The listing builds one solid part. Answer for the finished solid, in the listing's coordinates (mm). Face numbers are marked on the shaded views. A direction names the side the tool comes from. Give positions to 0.01 mm unless a question says otherwise; leave off trailing zeros. Write each loop counter-clockwise with the first axis right and the second up, starting at its lowest first coordinate (ties: lowest second). Pieces come first, ordered by that corner, then holes. Notation, with made-up numbers: (2, 62) - (23, 62) arc R23 cw to (23, 98) - close; hole circle Ø8 at (20.5, -23). An arc over 180 degrees is marked (long way). One line per question, with ' | ' between items. Start each with the question number.
1. A cutting plane is placed at D-D (z = 25.5). Determine the outline of the cut face in (x, y), then the cut area to 3 significant figures.
2. A cutting plane is placed at B-B (y = 40.5). Determine the outline of the cut face in (x, z).
3. Find the intervals of material crossed by L1, parallel to Y at x = 84.5, z = 9.5; L2, parallel to Y at x = 20.5, z = 34.5; L3, parallel to X at y = 16, z = 30, in increasing order. Write a range as from..to.
4. For the marked faces 1, 2 and 3, determine the directions among +Z, -Z, +X, -X, +Y, -Y from which every point of the face is accessible in a straight line to the end or side of a thin tool.
5. Given P1, Ø1, axis at x = 29, z = 10.5, coming from the -Y side, flat-ended and moving along its own axis, determine where the tip first touches the part or whether it passes through.
6. A cutting plane is placed at C-C (x = 132). Determine the outline of the cut face in (y, z).
7. The mould has two halves that part along X. Classify the marked faces 4, 5, 6 and 7: +X half, -X half, draft (parallel to the pull), parting line (faces both ways), or undercut.
8. A cutting plane is placed at A-A (x = 60). Determine the outline of the cut face in (y, z).
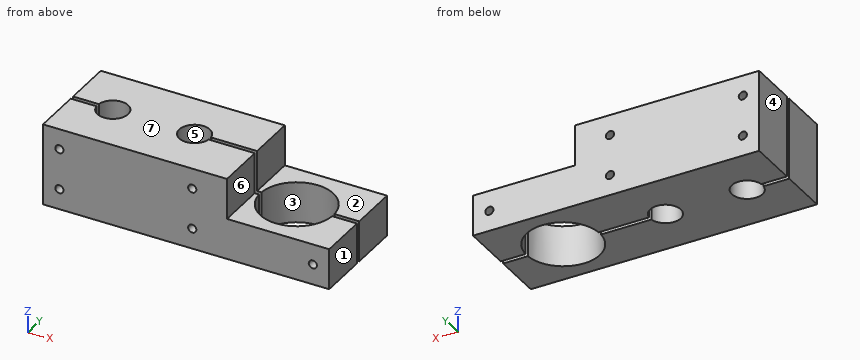
```python
from build123d import *

# Parameters (mm, degrees)
EXTRUDE_1_DEPTH     = 40
SKETCH_8_R          = 2
SKETCH_8_W          = 50
SKETCH_8_H          = 20
CUT_EXTRUDE_1_DEPTH = 50


with BuildPart() as part:
    # Эскиз1 → Бобышка-Вытянуть1 (new body)
    with BuildSketch(Plane.XY):
        with BuildLine():
            Line((67.432912675, 26.000904174), (92.128005404, 26.000904174))
            ThreePointArc((92.128005404, 26.000904174), (110, 42.9), (127.871994596, 26.000904174))
            Line((127.871994596, 26.000904174), (140, 26.000904174))
            Line((140, 26.000904174), (140, 50))
            Line((140, 50), (0, 50))
            Line((0, 50), (0, 26))
            Line((0, 26), (12.566965626, 26))
            ThreePointArc((12.566965626, 26), (27.5, 25), (12.566965626, 24))
            Line((12.566965626, 24), (0, 24))
            Line((0, 24), (0, 0))
            Line((0, 0), (140, 0))
            Line((140, 0), (140, 23.999095826))
            Line((140, 23.999095826), (127.871994596, 23.999095826))
            ThreePointArc((127.871994596, 23.999095826), (110, 7.1), (92.128005404, 23.999095826))
            Line((92.128005404, 23.999095826), (67.432912675, 23.999095826))
            ThreePointArc((67.432912675, 23.999095826), (52.5, 25), (67.432912675, 26.000904174))
        make_face()
    extrude(amount=EXTRUDE_1_DEPTH)

    # Эскиз8 → Вырез-Вытянуть1 (cut)
    with BuildSketch(Plane.XZ):
        with Locations(Location((8, 30, 0), (0, 0, 270))):
            Circle(SKETCH_8_R)
        with Locations(Location((8, 10, 0), (0, 0, 270))):
            Circle(SKETCH_8_R)
        with Locations(Location((132, 10, 0), (0, 0, 270))):
            Circle(SKETCH_8_R)
        with Locations(Location((73, 30, 0), (0, 0, 270))):
            Circle(SKETCH_8_R)
        with Locations(Location((73, 10, 0), (0, 0, 270))):
            Circle(SKETCH_8_R)
        with Locations((115, 30)):
            Rectangle(SKETCH_8_W, SKETCH_8_H)
    extrude(amount=-CUT_EXTRUDE_1_DEPTH, mode=Mode.SUBTRACT)


solid = part.part
```
Determined:
1) outline: (0, 0) - (90, 0) - (90, 24) - (67.43, 24) arc R7.5 cw (long way) to (67.43, 26) - (90, 26) - (90, 50) - (0, 50) - (0, 26) - (12.57, 26) arc R7.5 cw (long way) to (12.57, 24) - (0, 24) - close | area: 4,080 mm2
2) outline: (0, 0) - (101.05, 0) - (101.05, 20) - (90, 20) - (90, 40) - (0, 40) - close; (118.95, 0) - (140, 0) - (140, 20) - (118.95, 20) - close; hole circle Ø4 at (8, 10); hole circle Ø4 at (8, 30); hole circle Ø4 at (73, 10); hole circle Ø4 at (73, 30); hole circle Ø4 at (132, 10)
3) L1: 0..24, 26..50 | L2: 0..17.52, 32.48..50 | L3: 0..6, 10..71, 75..90
4) face 1: +Z, -Z, +X, +Y, -Y | face 2: +Z, +X, +Y, -Y | face 3: +Z, -Z
5) P1: y = 0
6) outline: (0, 0) - (24, 0) - (24, 8) - (0, 8) - close; (0, 12) - (24, 12) - (24, 20) - (0, 20) - close; (26, 0) - (50, 0) - (50, 8) - (26, 8) - close; (26, 12) - (50, 12) - (50, 20) - (26, 20) - close
7) face 4: -X half | face 5: undercut | face 6: +X half | face 7: draft
8) outline: (0, 0) - (17.5, 0) - (17.5, 40) - (0, 40) - close; (32.5, 0) - (50, 0) - (50, 40) - (32.5, 40) - close
